Work out the finished part from the listing and answer in its coordinate system (mm). A direction names the side the tool comes from. Coordinates: 2 decimals unless noted, no trailing zeros. Order: outer loops, then holes, each group sorted by start corner. A loop starts at its lowest first (then second) coordinate and runs counter-clockwise, first axis right, second up.
```python
from build123d import *

# Parameters (mm, degrees)
SKETCH_1_R          = 46.9
SKETCH_1_R_2        = 1.6
EXTRUDE_1_DEPTH     = 25
SKETCH_2_R          = 3
EXTRUDE_2_DEPTH     = 25
SKETCH_3_R          = 1.6
CUT_EXTRUDE_1_DEPTH = 71.881732484
CUT_EXTRUDE_2_DEPTH = 71.881732484
CUT_EXTRUDE_3_DEPTH = 69.296196254


with BuildPart() as part:
    # 草图1 → 凸台-拉伸1 (new body)
    with BuildSketch(Plane.XY):
        Circle(SKETCH_1_R)
        with Locations((12.835117837, 41.981778787)):
            Circle(SKETCH_1_R_2, mode=Mode.SUBTRACT)
        with Locations((-17.153096541, 40.410163067)):
            Circle(SKETCH_1_R_2, mode=Mode.SUBTRACT)
        with BuildLine():
            ThreePointArc((-17.670567057, 36.885783981), (5.183019571, -40.570263841), (7.829749303, 40.143555222))
            ThreePointArc((7.829749303, 40.143555222), (-5.183019571, 40.570263841), (-17.670567057, 36.885783981))
        make_face(mode=Mode.SUBTRACT)
    extrude(amount=EXTRUDE_1_DEPTH)

    # 草图2 → 凸台-拉伸2 (add)
    with BuildSketch(Plane.XY.offset(25)):
        with Locations((-31.749094475, 31.749094475)):
            Circle(SKETCH_2_R)
        with Locations((31.749094475, 31.749094475)):
            Circle(SKETCH_2_R)
        with Locations((31.749094475, -31.749094475)):
            Circle(SKETCH_2_R)
        with Locations((-31.749094475, -31.749094475)):
            Circle(SKETCH_2_R)
    extrude(amount=-EXTRUDE_2_DEPTH)

    # 草图3 → 切除-拉伸1 (cut, through all)
    with BuildSketch(Plane.XY.offset(25)):
        with Locations((-31.749094475, 31.749094475)):
            Circle(SKETCH_3_R)
        with Locations((-31.749094475, -31.749094475)):
            Circle(SKETCH_3_R)
        with Locations((31.749094475, -31.749094475)):
            Circle(SKETCH_3_R)
        with Locations((31.749094475, 31.749094475)):
            Circle(SKETCH_3_R)
    extrude(amount=-CUT_EXTRUDE_1_DEPTH, mode=Mode.SUBTRACT)

    # 草图4 → 切除-拉伸2 (cut, through all)
    with BuildSketch(Plane.XY.offset(25)):
        with BuildLine():
            ThreePointArc((-20.139957039, 40.129691383), (-19.72949951, 41.947091088), (-18.325289842, 43.171677663))
            ThreePointArc((-18.325289842, 43.171677663), (-25.271051352, 39.509289586), (-31.508446668, 34.739427004))
            ThreePointArc((-31.508446668, 34.739427004), (-30.445394472, 34.451013479), (-29.558090066, 33.798362559))
            ThreePointArc((-29.558090066, 33.798362559), (-25.049858336, 37.262777638), (-20.139957039, 40.129691383))
        make_face()
        with BuildLine():
            ThreePointArc((-14.876494449, 42.363898698), (-7.545559902, 44.261433842), (0, 44.9))
            Line((0, 44.9), (0, 46.9))
            ThreePointArc((0, 46.9), (-9.350356079, 45.958468656), (-18.325289842, 43.171677663))
            ThreePointArc((-18.325289842, 43.171677663), (-16.468950059, 43.331112158), (-14.876494449, 42.363898698))
        make_face()
        with BuildLine():
            ThreePointArc((31.508446668, 34.739427004), (23.168662113, 40.777727939), (13.712233545, 44.850692873))
            ThreePointArc((13.712233545, 44.850692873), (15.23675449, 43.779594513), (15.834933275, 42.015055494))
            ThreePointArc((15.834933275, 42.015055494), (23.065345276, 38.522718586), (29.558090066, 33.798362559))
            ThreePointArc((29.558090066, 33.798362559), (30.445394472, 34.451013479), (31.508446668, 34.739427004))
        make_face()
        with BuildLine():
            Line((0, 46.9), (0, 44.9))
            ThreePointArc((0, 44.9), (5.218754509, 44.595679178), (10.366766227, 43.686841932))
            ThreePointArc((10.366766227, 43.686841932), (11.849397199, 44.81521395), (13.712233545, 44.850692873))
            ThreePointArc((13.712233545, 44.850692873), (6.932261689, 46.384843946), (0, 46.9))
        make_face()
        with BuildLine():
            ThreePointArc((34.739427004, 31.508446668), (34.451013479, 30.445394472), (33.798362559, 29.558090066))
            ThreePointArc((33.798362559, 29.558090066), (44.9, 0), (33.798362559, -29.558090066))
            ThreePointArc((33.798362559, -29.558090066), (34.451013479, -30.445394472), (34.739427004, -31.508446668))
            ThreePointArc((34.739427004, -31.508446668), (46.9, 0), (34.739427004, 31.508446668))
        make_face()
        with BuildLine():
            ThreePointArc((31.508446668, -34.739427004), (30.445394472, -34.451013479), (29.558090066, -33.798362559))
            ThreePointArc((29.558090066, -33.798362559), (0, -44.9), (-29.558090066, -33.798362559))
            ThreePointArc((-29.558090066, -33.798362559), (-30.445394472, -34.451013479), (-31.508446668, -34.739427004))
            ThreePointArc((-31.508446668, -34.739427004), (0, -46.9), (31.508446668, -34.739427004))
        make_face()
        with BuildLine():
            ThreePointArc((-33.798362559, 29.558090066), (-44.9, 0), (-33.798362559, -29.558090066))
            ThreePointArc((-33.798362559, -29.558090066), (-34.451013479, -30.445394472), (-34.739427004, -31.508446668))
            ThreePointArc((-34.739427004, -31.508446668), (-46.9, 0), (-34.739427004, 31.508446668))
            ThreePointArc((-34.739427004, 31.508446668), (-34.451013479, 30.445394472), (-33.798362559, 29.558090066))
        make_face()
    extrude(amount=-CUT_EXTRUDE_2_DEPTH, mode=Mode.SUBTRACT)

    # 草图6 → 切除-拉伸3 (cut, through all)
    with BuildSketch(Plane(origin=(0, 0, 0), x_dir=(1, 0, 0), z_dir=(0, 1, 0))):
        with BuildLine():
            Line((-3.5, -3.5), (-3.5, 0))
            Line((-3.5, 0), (3.5, 0))
            Line((3.5, 0), (3.5, -3.5))
            ThreePointArc((3.5, -3.5), (0, -7), (-3.5, -3.5))
        make_face()
    extrude(amount=-CUT_EXTRUDE_3_DEPTH, mode=Mode.SUBTRACT)


solid = part.part
```
1. The part is cut by section C-C (z = 22.25). Determine the outline of the cut face in (x, y), plus the area to 3 significant figures.
2. The mould has two halves that part along X. Classify faces 1 (the cylindrical face through (-30.223, -31.268, 12.675)), 2 (the cylindrical face through (44.898, 0.452, 12.675)), 3 (the flat face through (40, 10, 0)): released by +X, released by -X, zero draft, split by the parting line, or undercut.
3. Flat-ended cylindrical pins translate along their axes: pin 1 (10 mm diameter, centred on x = -26, y = -19.5, fed in from +Z); pin 2 (3 mm diameter, centred on y = -18.5, z = 3, fed in from +X); pin 3 (5 mm diameter, centred on y = 4, z = 22, fed in from -X); pin 4 (2 mm diameter, centred on y = 6.5, z = 13, fed in from +X). Find the tip coordinate at first contact, or state that the pin passes through.
4. Consider probe 1 along X at (y, z) = (32.5, 15); probe 2 along Y at (x, z) = (30.5, 7.25); probe 3 along X at (y, z) = (0, 11.25). Determine where each line is inside the solid, lowest interval first.
5. For faces 4 (the flat face through (-3.5, -43, 2)), 5 (the cylindrical face through (-30.27, 31.14, 12.68)), determine the directions among +Z, -Z, +X, -X, +Y, -Y from which every point of the face is accessible in a straight line to the end or side of a thin tool.
6. The part is cut by section A-A (y = 0). Determine the outline of the cut face in (x, z), plus the area to 3 significant figures.
7. The part is cut by section B-B (x = 9). Determine the outline of the cut face in (y, z).
Worked out:
1. outline: (-33.8, -29.56) arc R3 ccw (long way) to (-29.56, -33.8) arc R44.9 ccw to (29.56, -33.8) arc R3 ccw (long way) to (33.8, -29.56) arc R44.9 ccw to (33.8, 29.56) arc R3 ccw (long way) to (29.56, 33.8) arc R44.9 ccw to (15.83, 42.02) arc R3 ccw to (10.37, 43.69) arc R44.9 ccw to (-14.88, 42.36) arc R3 ccw to (-20.14, 40.13) arc R44.9 ccw to (-29.56, 33.8) arc R3 ccw (long way) to (-33.8, 29.56) arc R44.9 ccw to start; hole circle Ø81.8 at (0, 0); hole circle Ø3.2 at (-31.75, -31.75); hole circle Ø3.2 at (-31.75, 31.75); hole circle Ø3.2 at (-17.15, 40.41); hole circle Ø3.2 at (12.84, 41.98); hole circle Ø3.2 at (31.75, -31.75); hole circle Ø3.2 at (31.75, 31.75)
1. area: 1,100 mm2
2. face 1: undercut
2. face 2: released by +X
2. face 3: zero draft
3. pin 1: passes through
3. pin 2: stops at x = 41.56
3. pin 3: stops at x = -44.87
3. pin 4: stops at x = 44.56
4. probe 1: x = -34.65 to -33.16, -30.34 to -24.83, 24.83 to 30.34, 33.16 to 34.65
4. probe 2: y = -34.48 to -32.75, -30.75 to -27.25, 27.25 to 30.75, 32.75 to 34.48
4. probe 3: x = -44.9 to -40.9, 40.9 to 44.9
5. face 4: -Z, -Y
5. face 5: +Z, -Z
6. outline: (-44.9, 0) - (-40.9, 0) - (-40.9, 25) - (-44.9, 25) - close; (40.9, 0) - (44.9, 0) - (44.9, 25) - (40.9, 25) - close
6. area: 200 mm2
7. outline: (-43.99, 0) - (-39.9, 0) - (-39.9, 25) - (-43.99, 25) - close; (39.9, 0) - (43.99, 0) - (43.99, 25) - (39.9, 25) - close
